```python
from build123d import *

# Parameters (mm, degrees)
ESBO_O7_R                = 2.5
RESSALTO_EXTRUS_O1_DEPTH = 5
ESBO_O8_R                = 2.5
RESSALTO_EXTRUS_O2_DEPTH = 5.5
ESBO_O9_R                = 1.5
CORTE_EXTRUS_O4_DEPTH    = 25
RESSALTO_EXTRUS_O3_START = 5
RESSALTO_EXTRUS_O3_DEPTH = 5
CORTE_EXTRUS_O5_DEPTH    = 16
SKETCH1_R                = 3.5
SKETCH1_R_2              = 2.5
BOSS_EXTRUDE1_DEPTH      = 0.5


with BuildPart() as part:
    # Esboço7 → Ressalto-extrusão1 (new body)
    with BuildSketch(Plane.XY):
        with BuildLine():
            Line((6, 0), (6, -12))
            ThreePointArc((6, -12), (0, -18), (-6, -12))
            Line((-6, -12), (-6, -10.710094321))
            ThreePointArc((-6, -10.710094321), (-6.452901427, -9.873026133), (-7.401366303, -9.794176699))
            Line((-7.401366303, -9.794176699), (-41.221941829, -24.614766505))
            ThreePointArc((-41.221941829, -24.614766505), (-45.173793605, -23.071112549), (-46.717447562, -27.022964325))
            Line((-46.717447562, -27.022964325), (-52.212953295, -29.431162145))
            ThreePointArc((-52.212953295, -29.431162145), (-52.399466586, -20.248653784), (-46.038337469, -13.62375504))
            Line((-46.038337469, -13.62375504), (-2.40819782, 5.495505733))
            ThreePointArc((-2.40819782, 5.495505733), (3.282591437, 5.022409129), (6, 0))
        make_face()
        Circle(ESBO_O7_R, mode=Mode.SUBTRACT)
    extrude(amount=RESSALTO_EXTRUS_O1_DEPTH)

    # Esboço8 → Ressalto-extrusão2 (add)
    with BuildSketch(Plane(origin=(0, 0, 0), x_dir=(-1, 0, 0), z_dir=(0, 0, -1))):
        with Locations(Location((0, -12, 0), (0, 0, 180))):
            Circle(ESBO_O8_R)
    extrude(amount=RESSALTO_EXTRUS_O2_DEPTH)

    # Esboço9 → Corte-extrusão4 (cut)
    with BuildSketch(Plane(origin=(0, 0, -5.5), x_dir=(-1, 0, 0), z_dir=(0, 0, -1))):
        with Locations((0, -12)):
            Circle(ESBO_O9_R)
    extrude(amount=-CORTE_EXTRUS_O4_DEPTH, mode=Mode.SUBTRACT)

    # Esboço10 → Ressalto-extrusão3 (add)
    with BuildSketch(Plane(origin=(0, 0, 0), x_dir=(-1, 0, 0), z_dir=(0, 0, -1)).offset(RESSALTO_EXTRUS_O3_START)):
        with BuildLine():
            Line((46.717447562, -27.022964325), (52.212953295, -29.431162145))
            ThreePointArc((52.212953295, -29.431162145), (46.038337469, -13.62375504), (30.230930363, -19.798370866))
            Line((30.230930363, -19.798370866), (41.221941829, -24.614766505))
            ThreePointArc((41.221941829, -24.614766505), (45.173793605, -23.071112549), (46.717447562, -27.022964325))
        make_face()
    extrude(amount=-RESSALTO_EXTRUS_O3_DEPTH)

    # Esboço11 → Corte-extrusão5 (cut)
    with BuildSketch(Plane(origin=(-2.40819782, 5.495505733, 0), x_dir=(-0.9159176221486778, -0.40136630331595097, 0), z_dir=(-0.40136630331595097, 0.9159176221486778, 0))):
        with BuildLine():
            Line((47.63544078, 2), (53.63544078, 2))
            ThreePointArc((53.63544078, 2), (55.63544078, 0), (53.63544078, -2))
            Line((53.63544078, -2), (47.63544078, -2))
            ThreePointArc((47.63544078, -2), (45.63544078, 0), (47.63544078, 2))
        make_face()
    extrude(amount=-CORTE_EXTRUS_O5_DEPTH, mode=Mode.SUBTRACT)

    # Sketch1 → Boss-Extrude1 (add)
    with BuildSketch(Plane(origin=(0, 0, 0), x_dir=(-1, 0, 0), z_dir=(0, 0, -1))):
        with Locations(Location((0, -12, 0), (0, 0, 180))):
            Circle(SKETCH1_R)
        with Locations((0, -12)):
            Circle(SKETCH1_R_2, mode=Mode.SUBTRACT)
    extrude(amount=BOSS_EXTRUDE1_DEPTH)


solid = part.part
```
Design review of the part built by this model. Coordinates are the model's own, in mm. A direction names the side the tool comes from. Give positions to 0.01 mm unless a question says otherwise; leave off trailing zeros. Order: outer loops, then holes, each group sorted by start corner. A loop starts at its lowest first (then second) coordinate and runs counter-clockwise, first axis right, second up. Notation, with made-up numbers: (55.5, 45.25) - (69.5, 45.25) arc R30 ccw to (69.5, 69.25) - close; hole circle Ø7 at (62, 67.25). An arc over 180 degrees is marked (long way). Use a Markdown table: item, result. Add a question column.
(1) Machinability: for faces 1 (the face through (-47, -19, -2)), 2 (the face through (-6, -11, 2)), 3 (the face through (-41.832, -18.24, -0.044)), which of the approach directions +Z, -Z, +X, -X, +Y, -Y give a long, thin tool a straight path to every point of the face, cutting with its end or side? Answer none if there is none.
(2) Add section A-A on x = 0. Give the boundary of the cut face in (y, z).
(3) Add section D-D on z = 3.75. Give the boundary of the cut face in (x, y).
(4) Wall thickness on probe 1 along Y at (x, z) = (0, 3.2); probe 2 along Y at (x, z) = (0, -2.25); probe 3 along X at (y, z) = (-12.5, 2.5): over which ranges is each line inside the solid? List them lowest first. Write a range as [from, to].
(5) Add section C-C on z = 1.25. Give the boundary of the cut face in (x, y), then the cut area to 3 significant figures.
(6) Mouldability with a two-part tool opening along X and no side actions: class faces 4 (the face through (3.21, 5.07, 2.46)), 5 (the face through (6, -6, 2)), 6 (the face through (-0.759, -8.583, -0.246)) as +X half, -X half, draft (parallel to the pull), parting line (faces both ways), or undercut.
(7) Clearance check with flat-ended pins moving along their axes: P1, Ø18.5, axis at x = -39, y = -23, coming from the -Z side; P2, Ø4, axis at x = -18, y = -11, coming from the -Z side. State where each tip first meets the part, or that it passes through.
Report:
| question | item | result |
|---|---|---|
| 1 | face 1 | none |
| 1 | face 2 | +Z, -Z, -Y |
| 1 | face 3 | -Y |
| 2 | outline | (-18, 0) - (-15.5, 0) - (-15.5, -0.5) - (-14.5, -0.5) - (-14.5, -5.5) - (-13.5, -5.5) - (-13.5, 5) - (-18, 5) - close; (-10.5, -5.5) - (-9.5, -5.5) - (-9.5, -0.5) - (-8.5, -0.5) - (-8.5, 0) - (-2.5, 0) - (-2.5, 5) - (-10.5, 5) - close; (2.5, 0) - (6, 0) - (6, 5) - (2.5, 5) - close |
| 3 | outline | (-52.21, -29.43) - (-46.72, -27.02) arc R3 cw to (-41.22, -24.61) - (-7.4, -9.79) arc R1 cw to (-6, -10.71) - (-6, -12) arc R6 ccw to (6, -12) - (6, 0) arc R6 ccw to (-2.41, 5.5) - (-46.04, -13.62) arc R12 ccw to start; hole circle Ø5 at (0, 0); hole circle Ø3 at (0, -12) |
| 4 | probe 1 | y = [-18, -13.5], [-10.5, -2.5], [2.5, 6] |
| 4 | probe 2 | y = [-14.5, -13.5], [-10.5, -9.5] |
| 4 | probe 3 | x = [-43.47, -13.58], [-5.98, -1.41], [1.41, 5.98] |
| 5 | outline | (-52.21, -29.43) - (-48.15, -27.65) - (-51.89, -19.11) arc R12 ccw to start; (-44.61, -13) - (-39.79, -23.99) - (-7.4, -9.79) arc R1 cw to (-6, -10.71) - (-6, -12) arc R6 ccw to (6, -12) - (6, 0) arc R6 ccw to (-2.41, 5.5) - close; hole circle Ø5 at (0, 0); hole circle Ø3 at (0, -12) |
| 5 | area | 737 mm² |
| 6 | face 4 | parting line |
| 6 | face 5 | +X half |
| 6 | face 6 | undercut |
| 7 | P1 | stops at z = -5 |
| 7 | P2 | stops at z = 0 |
